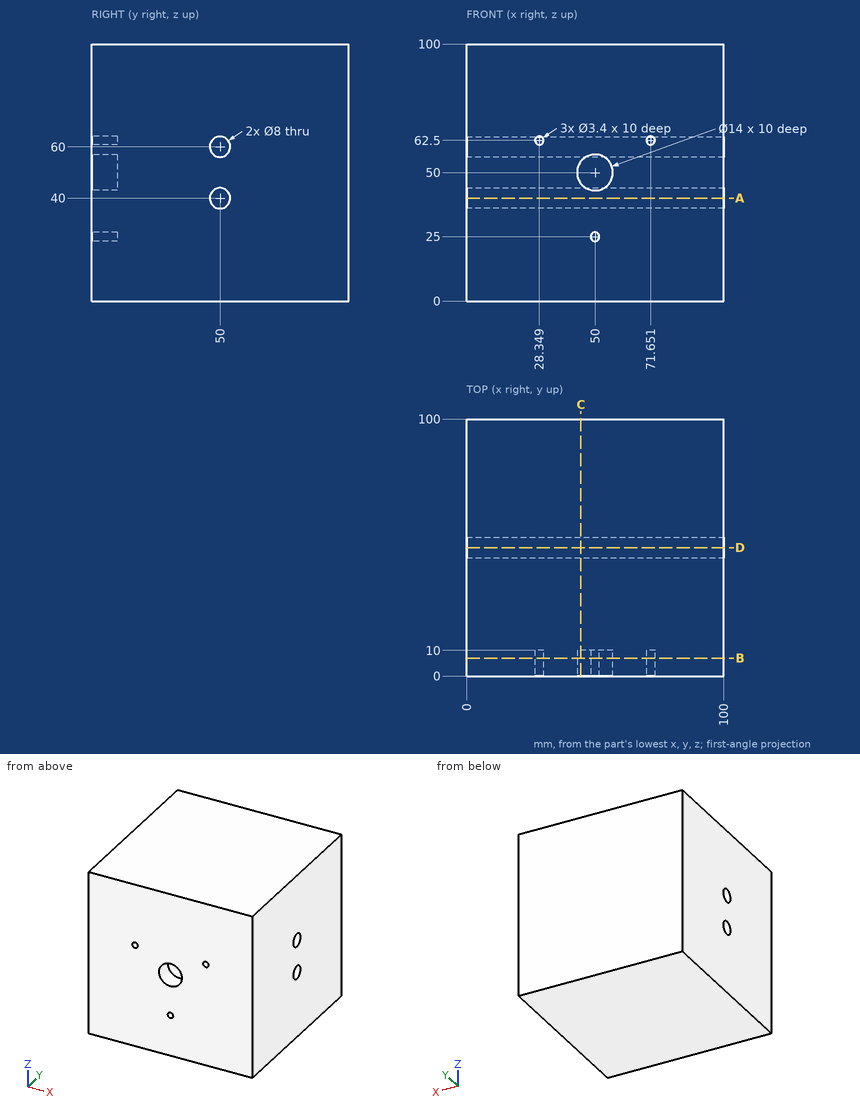
Source: three-view drawing plus pictorial views. Frame: mm from the lowest corner of the part. Give positions to 0.01 mm unless a question says otherwise; leave off trailing zeros. Write each loop counter-clockwise with the first axis right and the second up, starting at its lowest first coordinate (ties: lowest second). Pieces come first, ordered by that corner, then holes. Notation, with made-up numbers: (-2.75, 87.25) -> (44.25, 87.25) arc R35 cw to (44.25, 123.25) -> close; hole circle Ø5 at (84, 7.5). An arc over 180 degrees is marked (long way). Write item = value, one per line.
Q1. Cut plane C-C on x = 44.5. Return loops of the section in (y, z), then the cut area to 3 significant figures.
Here are the results:
outline = (0, 0) -> (100, 0) -> (100, 100) -> (0, 100) -> (0, 54.33) -> (10, 54.33) -> (10, 45.67) -> (0, 45.67) -> close; hole circle Ø8 at (50, 40); hole circle Ø8 at (50, 60)
area = 9,810 mm²
Q2. Cut plane A-A on z = 40. Return loops of the section in (x, y), then the cut area to 3 significant figures.
Here are the results:
outline = (0, 0) -> (100, 0) -> (100, 46) -> (0, 46) -> close; (0, 54) -> (100, 54) -> (100, 100) -> (0, 100) -> close
area = 9,200 mm²
Q3. Line query: line 1 (Z direction, x = 50, y = 7.5); line 2 (Y direction, x = 42, z = 60); line 3 (Z direction, x = 42, y = 48) (1 decimal). Output: solid intervals per line, ascending. Write a range as from..to.
Here are the results:
line_1 = 0..23.3, 26.7..43, 57..100
line_2 = 0..46, 54..100
line_3 = 0..36.5, 43.5..56.5, 63.5..100
Q4. First-contact query: pin 1 (1 mm diameter, centred on x = 71, z = 62.5, fed in from -Y); pin 2 (7 mm diameter, centred on y = 50, z = 40, fed in from -X). Flat tips, straight axial feed; report the tip coordinate or a pass-through.
Here are the results:
pin_1 = 10
pin_2 = through
Q5. Cut plane B-B on y = 7. Return loops of the section in (x, z).
Here are the results:
outline = (0, 0) -> (100, 0) -> (100, 100) -> (0, 100) -> close; hole circle Ø3.4 at (28.35, 62.5); hole circle Ø14 at (50, 50); hole circle Ø3.4 at (50, 25); hole circle Ø3.4 at (71.65, 62.5)
Q6. Cut plane D-D on y = 50. Return loops of the section in (x, z), then the cut area to 3 significant figures.
Here are the results:
outline = (0, 0) -> (100, 0) -> (100, 36) -> (0, 36) -> close; (0, 44) -> (100, 44) -> (100, 56) -> (0, 56) -> close; (0, 64) -> (100, 64) -> (100, 100) -> (0, 100) -> close
area = 8,400 mm²
